```python
from build123d import *

# Parameters (mm, degrees)
F1_DEPTH = 5


with BuildPart() as f1:
    # F0 (on Front) → F1 (new body)
    with BuildSketch(Plane.XZ):
        Polygon((0, 5), (0, 0), (2.817796, 0), (0.656805, 1.247649), (0.656805, 3.747649), (2.821869, 4.997649), (4.986932, 3.747649), (4.986932, 1.247649), (2.825941, 0), (16, 0), (16, 5), (13.399874, 5), (15.50617, 3.78393), (15.50617, 1.28393), (13.341106, 0.03393), (11.176043, 1.28393), (11.176043, 3.78393), (13.282339, 5), (8.131277, 5), (10.282767, 3.757837), (10.282767, 1.257837), (8.117704, 0.007837), (5.95264, 1.257837), (5.95264, 3.757837), (8.10413, 5), align=None)
    extrude(amount=F1_DEPTH)


solid = f1.part
```
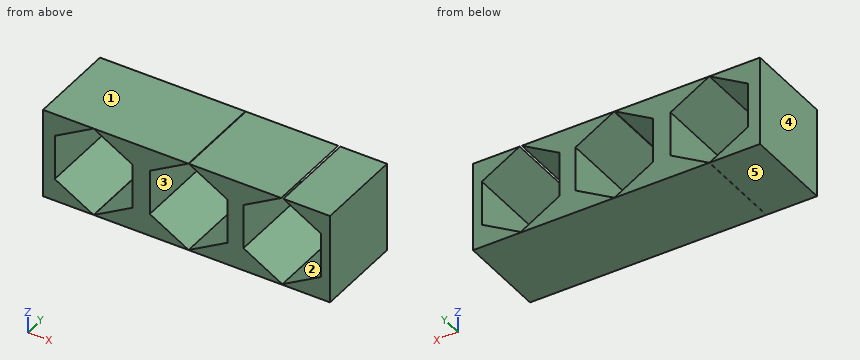
Can you work these out from the model? Positions are in its coordinate system, mm. Face numbers are marked on the shaded views. A direction names the side the tool comes from. Coordinates: 2 decimals unless noted, no trailing zeros. Order: outer loops, then holes, each group sorted by start corner. A loop starts at its lowest first (then second) coordinate and runs counter-clockwise, first axis right, second up. Notation, with made-up numbers: (17, -22) -> (75, -22) arc R16 cw to (75, -2) -> close; hole circle Ø7 at (74, -31). An arc over 180 degrees is marked (long way). Write each question's results on one line, items separated by ' | '.
Item 1: I want a section at D-D, the plane z = 0.8. Write out the boundary of the cut face in (x, y), then the cut area to 3 significant figures.
Results are:
outline: (0, -5) -> (1.43, -5) -> (1.43, 0) -> (0, 0) -> close; (4.21, -5) -> (6.75, -5) -> (6.75, 0) -> (4.21, 0) -> close; (9.49, -5) -> (12.01, -5) -> (12.01, 0) -> (9.49, 0) -> close; (14.67, -5) -> (16, -5) -> (16, 0) -> (14.67, 0) -> close | area: 39.1 mm²
Item 2: Which directions (+Z, -Z, +X, -X, +Y, -Y) give clear straight access to the entire face, cutting with the end or side of a thin tool? Please do the marked faces 1 and 2.
Results are:
face 1: +Z, +X, -X, +Y, -Y | face 2: +Y, -Y
Item 3: I want a section at B-B, the plane x = 2.5. Write out the boundary of the cut face in (y, z).
Results are:
outline: (-5, 0) -> (0, 0) -> (0, 0.18) -> (-5, 0.18) -> close; (-5, 4.81) -> (0, 4.81) -> (0, 5) -> (-5, 5) -> close
Item 4: If I drill on line 1 along X through (y, z) = (-3.4, 3.45); line 2 along X through (y, z) = (-1.4, 0.7); line 3 along Z through (x, y) = (2.5, -3.55), over which ranges is the centre line in solid material (lowest first)?
Results are:
line 1: 0 to 0.66, 4.99 to 5.95, 10.28 to 11.18, 15.51 to 16 | line 2: 0 to 1.61, 4.04 to 6.92, 9.32 to 12.19, 14.49 to 16 | line 3: 0 to 0.18, 4.81 to 5
Item 5: If we mould it in two halves opening along X, with no side actions, what happens to the marked faces 3, 4 and 5? For each: +X half, -X half, draft (parallel to the pull), parting line (faces both ways), or undercut.
Results are:
face 3: undercut | face 4: -X half | face 5: draft
Item 6: I want a section at A-A, the plane z = 1.7. Write out the boundary of the cut face in (x, y).
Results are:
outline: (0, -5) -> (0.66, -5) -> (0.66, 0) -> (0, 0) -> close; (4.99, -5) -> (5.95, -5) -> (5.95, 0) -> (4.99, 0) -> close; (10.28, -5) -> (11.18, -5) -> (11.18, 0) -> (10.28, 0) -> close; (15.51, -5) -> (16, -5) -> (16, 0) -> (15.51, 0) -> close
Item 7: I want a section at C-C, the plane y = -1. Write out the boundary of the cut face in (x, z).
Results are:
outline: (0, 0) -> (2.82, 0) -> (0.66, 1.25) -> (0.66, 3.75) -> (2.82, 5) -> (4.99, 3.75) -> (4.99, 1.25) -> (2.83, 0) -> (16, 0) -> (16, 5) -> (13.4, 5) -> (15.51, 3.78) -> (15.51, 1.28) -> (13.34, 0.03) -> (11.18, 1.28) -> (11.18, 3.78) -> (13.28, 5) -> (8.13, 5) -> (10.28, 3.76) -> (10.28, 1.26) -> (8.12, 0.01) -> (5.95, 1.26) -> (5.95, 3.76) -> (8.1, 5) -> (0, 5) -> close
